CAD build for the part. Positions are in the model's coordinates, mm. A direction names the side the tool comes from. Coordinates: 2 decimals unless noted, no trailing zeros. Loops run counter-clockwise (first coordinate to the right, second up) from the corner with the lowest first, then second, coordinate; pieces in that order, holes last.
1) Saw through at B-B, the plane x = 182. Write the cut outline in (y, z).
2) Pin check, flat tip, straight feed: pin 1 Ø2 at (x, y) = (180, -4.5) entering from +Z. Stop position of the tip, or through.
3) Which spindle directions (+Z, -Z, +X, -X, +Y, -Y) get a long thin tool onto all of the face, cutting with end or side? Do faces 4 (the flat face through (196.5, 0, 30)), 5 (the flat face through (-295, 0, 54.3)). Say none if no direction does.
4) Wall check: line 1 along X through (y, z) = (-4.25, 46) (3 decimals); line 2 along X through (y, z) = (0, 4) (3 decimals); line 3 along Z through (x, y) = (-218, 3.5). Give the ranges that are in metal, low to high.
5) Saw through at A-A, the plane y = -4.5. Write the cut outline in (x, z) (3 decimals), and give its area (3 significant figures).
6) Two-plate mould, pull along X, no slides. Class faces 1 (the flat face through (-226, 0, 2.7)), 2 (the flat face through (342.875, 0, 1)), 3 (the flat face through (-24, 0, 54.3)): +X half, -X half, draft (parallel to the pull), parting line (faces both ways), or undercut.
```python
from build123d import *

# Parameters (mm, degrees)
F0_W     = 342.875
F0_H     = 15
F1_DEPTH = 54.3
F4_DEPTH = 15


with BuildPart() as f1:
    # F0 (on Top) → F1 (new body, symmetric)
    with BuildSketch(Plane.XY):
        with Locations((171.4375, 0)):
            Rectangle(F0_W, F0_H)
    extrude(amount=F1_DEPTH, both=True)

    # F2: F1 across face


with BuildPart() as f1_1:
    add(f1.part)
    add(f1.part.mirror(Plane(origin=(0, 0, 0), x_dir=(0, -1, 0), z_dir=(-1, 0, 0))))

    # F3 (on face) → F4 (cut, through all)
    with BuildSketch(Plane(origin=(0, 7.5, 0), x_dir=(-1, 0, 0), z_dir=(0, 1, 0))):
        with BuildLine():
            Line((-151.5, 54.3), (-196.5, 54.3))
            Line((-196.5, 54.3), (-196.5, 5.7))
            ThreePointArc((-196.5, 5.7), (-195.62132, 3.57868), (-193.5, 2.7))
            Line((-193.5, 2.7), (-154.5, 2.7))
            ThreePointArc((-154.5, 2.7), (-152.37868, 3.57868), (-151.5, 5.7))
            Line((-151.5, 5.7), (-151.5, 54.3))
        make_face()
        with BuildLine():
            Line((248.5, 54.3), (203.5, 54.3))
            Line((203.5, 54.3), (203.5, 5.7))
            ThreePointArc((203.5, 5.7), (204.37868, 3.57868), (206.5, 2.7))
            Line((206.5, 2.7), (245.5, 2.7))
            ThreePointArc((245.5, 2.7), (247.62132, 3.57868), (248.5, 5.7))
            Line((248.5, 5.7), (248.5, 54.3))
        make_face()
    extrude(amount=-F4_DEPTH, mode=Mode.SUBTRACT)


solid = f1_1.part
```
Data:
1. outline: (-7.5, -54.3) - (7.5, -54.3) - (7.5, 2.7) - (-7.5, 2.7) - close
2. pin 1: stops at z = 2.7
3. face 4: +Z, +Y, -Y
3. face 5: +Z, +X, -X, +Y, -Y
4. line 1: x = -342.875 to -248.5, -203.5 to 151.5, 196.5 to 342.875
4. line 2: x = -342.875 to -247.972, -204.028 to 152.028, 195.972 to 342.875
4. line 3: z = -54.3 to 2.7
5. outline: (-342.875, -54.3) - (342.875, -54.3) - (342.875, 54.3) - (196.5, 54.3) - (196.5, 5.7) arc R3 cw to (193.5, 2.7) - (154.5, 2.7) arc R3 cw to (151.5, 5.7) - (151.5, 54.3) - (-203.5, 54.3) - (-203.5, 5.7) arc R3 cw to (-206.5, 2.7) - (-245.5, 2.7) arc R3 cw to (-248.5, 5.7) - (-248.5, 54.3) - (-342.875, 54.3) - close
5. area: 69,800 mm2
6. face 1: undercut
6. face 2: +X half
6. face 3: draft
